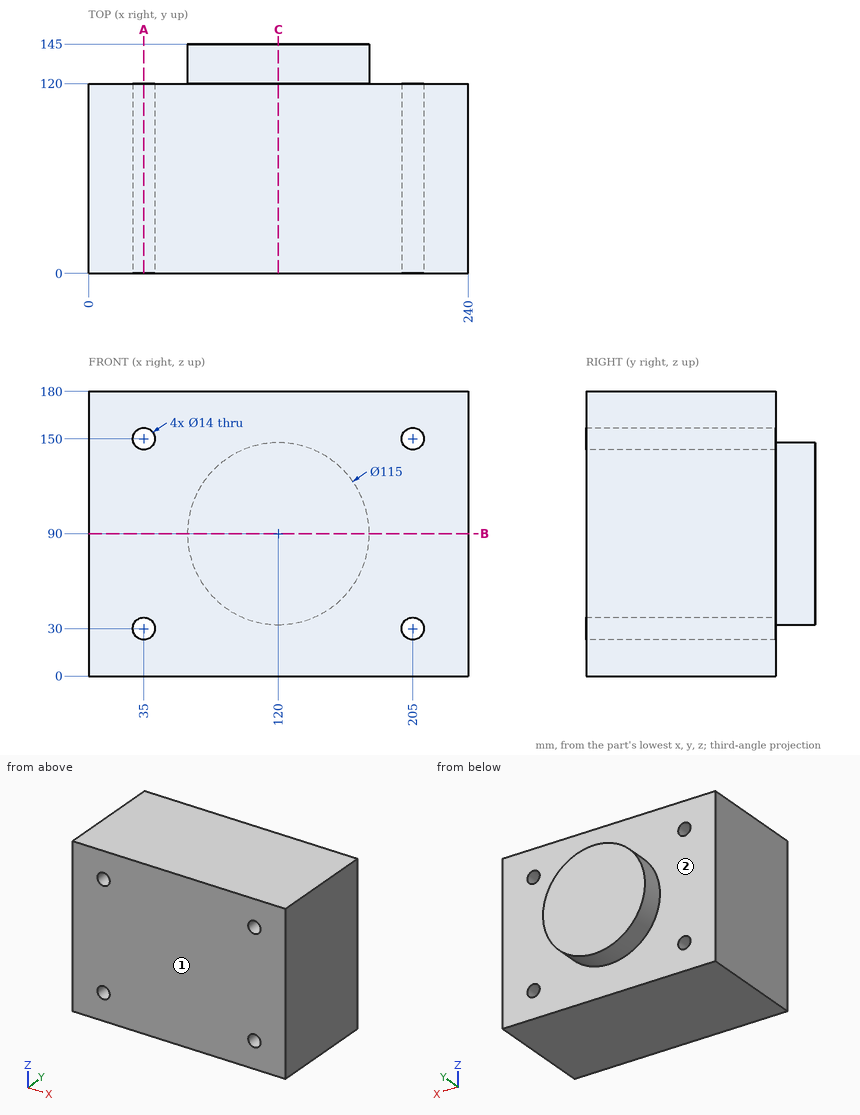
Study the drawing (mm; zero at the part's minimum x, y, z) and answer. A direction names the side the tool comes from. Give positions to 0.01 mm unless a question says otherwise; leave off trailing zeros. Write each loop counter-clockwise with the first axis right and the second up, starting at its lowest first coordinate (ties: lowest second). Pieces come first, ordered by that corner, then holes. Notation, with made-up numbers: (78, 73.5) -> (101, 73.5) arc R21 ccw to (101, 84.5) -> close; hole circle Ø3 at (5.5, -30.5). An arc over 180 degrees is marked (long way). Write item = value, one per line.
Q1. Section B-B on z = 90 is taken. Determine the outline of the cut face in (x, y), and give its area (3 significant figures).
Computed values:
outline = (0, 0) -> (240, 0) -> (240, 120) -> (177.5, 120) -> (177.5, 145) -> (62.5, 145) -> (62.5, 120) -> (0, 120) -> close
area = 31,700 mm^2
Q2. Flat-ended cylindrical pins translate along their axes: pin 1 Ø10 at (x, y) = (129.5, 128) entering from +Z; pin 2 Ø22.5 at (x, z) = (205, 150) entering from +Y. Find the tip coordinate at first contact, or state that the pin passes through.
Computed values:
pin_1 = 147.32
pin_2 = 120
Q3. Consider line 1 along X through (y, z) = (69.5, 30); line 2 along Y through (x, z) = (204, 52.5); line 3 along X through (y, z) = (14, 149). Determine where each line is inside the solid, lowest interval first.
Computed values:
line_1 = 0 to 28, 42 to 198, 212 to 240
line_2 = 0 to 120
line_3 = 0 to 28.07, 41.93 to 198.07, 211.93 to 240
Q4. Section C-C on x = 120 is taken. Determine the outline of the cut face in (y, z).
Computed values:
outline = (0, 0) -> (120, 0) -> (120, 32.5) -> (145, 32.5) -> (145, 147.5) -> (120, 147.5) -> (120, 180) -> (0, 180) -> close
Q5. A tool of negligible diameter and unlimited length cuts with its end or side. For the marked faces 1 and 2, from which of +Z, -Z, +X, -X, +Y, -Y can it reach the whole face along a straight path? Write none if from no direction.
Computed values:
face_1 = +Z, -Z, +X, -X, -Y
face_2 = +Y
Q6. Section A-A on x = 35 is taken. Determine the outline of the cut face in (y, z), and give its area (3 significant figures).
Computed values:
outline = (0, 0) -> (120, 0) -> (120, 23) -> (0, 23) -> close; (0, 37) -> (120, 37) -> (120, 143) -> (0, 143) -> close; (0, 157) -> (120, 157) -> (120, 180) -> (0, 180) -> close
area = 18,200 mm^2
